```python
from build123d import *

# Parameters (mm, degrees)
SKETCH1_W          = 15
SKETCH1_H          = 9
BASE_FLANGE1_DEPTH = 0.7
EDGE_FLANGE1_DEPTH = 15
CUT_EXTRUDE1_DEPTH = 10
FILLET1_R          = 2
CUT_EXTRUDE2_DEPTH = 10


# Sheet-metal steps are written as plain solids
with BuildPart() as part:
    # Sketch1 → Base-Flange1 (new body)
    with BuildSketch(Plane(origin=(0, 0, 0), x_dir=(1, 0, 0), z_dir=(0, 1, 0))):
        with Locations((7.5, -4.5)):
            Rectangle(SKETCH1_W, SKETCH1_H)
    extrude(amount=-BASE_FLANGE1_DEPTH)

    # Edge-Flange1 section (across the edge) → Edge-Flange1 (add)
    with BuildSketch(Plane(origin=(0, 0, 9.7366), x_dir=(0, 0, -1), z_dir=(1, 0, 0))):
        with BuildLine():
            Line((-0.7, 0.7366), (-0.7, 15))
            Line((-0.7, 15), (0, 15))
            Line((0, 15), (0, 0.7366))
            ThreePointArc((0, 0.7366), (0.215745145, 0.215745145), (0.7366, 0))
            Line((0.7366, 0), (0.7366, -0.7))
            ThreePointArc((0.7366, -0.7), (-0.279229602, -0.279229602), (-0.7, 0.7366))
        make_face()
    extrude(amount=EDGE_FLANGE1_DEPTH)

    # Sketch7 → Cut-Extrude1 (cut)
    with BuildSketch(Plane(origin=(0, 0, 0), x_dir=(1, 0, 0), z_dir=(0, 1, 0))):
        with BuildLine():
            Line((8.5, -5.2), (6.5, -5.2))
            ThreePointArc((6.5, -5.2), (4.8, -3.5), (6.5, -1.8))
            Line((6.5, -1.8), (8.5, -1.8))
            ThreePointArc((8.5, -1.8), (10.2, -3.5), (8.5, -5.2))
        make_face()
    extrude(amount=-CUT_EXTRUDE1_DEPTH, mode=Mode.SUBTRACT)

    # Fillet1
    fillet1_edges = [part.edges().sort_by_distance(p)[0] for p in [
        (0, 15, 10.0866),
        (15, 15, 10.0866),
        (0, -0.35, 0),
        (15, -0.35, 0),
    ]]
    fillet(fillet1_edges, radius=FILLET1_R)

    # Sketch8 → Cut-Extrude2 (cut)
    with BuildSketch(Plane(origin=(0, 0, 9.7366), x_dir=(-1, 0, 0), z_dir=(0, 0, -1))):
        with BuildLine():
            Line((-5.8, 12), (-5.8, 8))
            ThreePointArc((-5.8, 8), (-7.5, 6.3), (-9.2, 8))
            Line((-9.2, 8), (-9.2, 12))
            ThreePointArc((-9.2, 12), (-7.5, 13.7), (-5.8, 12))
        make_face()
    extrude(amount=-CUT_EXTRUDE2_DEPTH, mode=Mode.SUBTRACT)


solid = part.part
```
Here's how the part is built. I have some questions about the finished solid (model axes, mm). A direction names the side the tool comes from. Round coordinates to 2 decimals unless told otherwise and drop trailing zeros. Loops run counter-clockwise (first coordinate to the right, second up) from the corner with the lowest first, then second, coordinate; pieces in that order, holes last.
1. Suppose I cut it at A-A, the plane z = 3.5. Please give me the cut outline in (x, y).
Answers:
outline: (0, -0.7) - (4.8, -0.7) - (4.8, 0) - (0, 0) - close; (10.2, -0.7) - (15, -0.7) - (15, 0) - (10.2, 0) - close
2. For faces 1 (the face through (7.4, 0, 5.4)), 2 (the face through (4.8, -0.3, 3.5)), 3 (the face through (7.5, 6.3, 10.1)), which set-ups out of +Z, -Z, +X, -X, +Y, -Y let a thin tool reach every point of the face, with its end or its side?
Answers:
face 1: -Z, +X, -X, +Y
face 2: +Y, -Y
face 3: +Z, -Z
3. Thinking about a two-plate mould opening in X: for faces 4 (the face through (10.2, -0.3, 3.5)), 5 (the face through (6, 6, 9.737)), 6 (the face through (0.57, -0.35, 0.6)), which applies, released by +X, released by -X, zero draft, split by the parting line, or undercut?
Answers:
face 4: undercut
face 5: zero draft
face 6: released by -X
4. Suppose I cut it at C-C, the plane x = 2.25. Please give me the cut outline in (y, z), and give its area (3 significant figures).
Answers:
outline: (-0.7, 0) - (0, 0) - (0, 9) arc R0.74 cw to (0.74, 9.74) - (15, 9.74) - (15, 10.44) - (0.74, 10.44) arc R1.44 ccw to (-0.7, 9) - close
area: 17.5 mm2
5. If I drill on probe 1 along Y at (x, z) = (6.25, 7.25); probe 2 along Z at (x, y) = (9, 14.25), over which ranges is the centre line in solid material (lowest first)?
Answers:
probe 1: y = -0.7 to 0
probe 2: z = 9.74 to 10.44
6. Suppose I cut it at B-B, the plane y = 8.25. Please give me the cut outline in (x, z), and give its area (3 significant figures).
Answers:
outline: (0, 9.74) - (5.8, 9.74) - (5.8, 10.44) - (0, 10.44) - close; (9.2, 9.74) - (15, 9.74) - (15, 10.44) - (9.2, 10.44) - close
area: 8.12 mm2
7. Suppose I cut it at D-D, the plane x = 6.25. Please give me the cut outline in (y, z).
Answers:
outline: (-0.7, 0) - (0, 0) - (0, 1.82) - (-0.7, 1.82) - close; (-0.7, 5.18) - (0, 5.18) - (0, 9) arc R0.74 cw to (0.74, 9.74) - (6.85, 9.74) - (6.85, 10.44) - (0.74, 10.44) arc R1.44 ccw to (-0.7, 9) - close; (13.15, 9.74) - (15, 9.74) - (15, 10.44) - (13.15, 10.44) - close
8. Will these pins go through, and if not, where does the flat tip stop? pin 1 (6 mm diameter, centred on y = 4, z = 6, fed in from +X); pin 2 (3 mm diameter, centred on x = 3, z = 5, fed in from +Y); pin 3 (0.8 mm diameter, centred on x = 7, y = -0.5, fed in from +Z).
Answers:
pin 1: passes through
pin 2: stops at y = 0
pin 3: stops at z = 10.17
